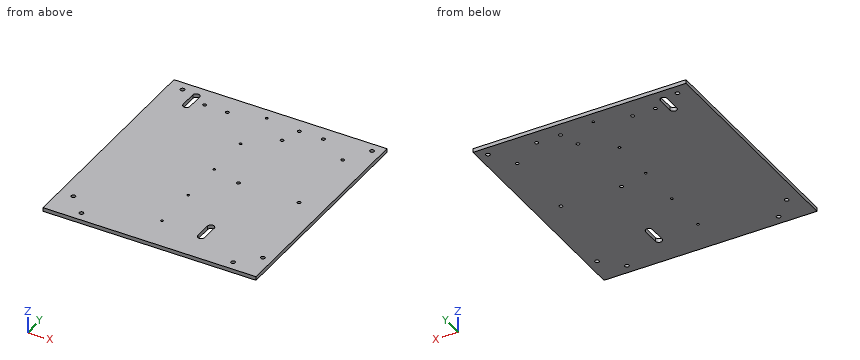
Autodesk Inventor part; units mm, degrees
ref_plane "YZ Plane" through (0, 0, 0) normal (1, 0, 0) x (0, 1, 0)
ref_plane "XZ Plane" through (0, 0, 0) normal (0, 1, 0) x (-1, 0, 0)
ref_plane "XY Plane" through (0, 0, 0) normal (0, 0, 1) x (1, 0, 0)
sketch "Sketch1" plane through (0, 0, 0) normal (0, 0, 1) x (1, 0, 0)
  line L0 (-140.5, -150) -> (140.5, -150)
  line L1 (140.5, -150) -> (140.5, 150)
  line L2 (140.5, 150) -> (-140.5, 150)
  line L3 (-140.5, 150) -> (-140.5, -150)
  line L4 (-140.5, -150) -> (140.5, 150) construction
  line L5 (140.5, -150) -> (-140.5, 150) construction
  point P0 (0, 0)
  dimension "d0" = 300
  dimension "d1" = 281
extrude "Extrusion1" add sketch "Sketch1" along normal blind 5
sketch "Sketch5" plane through (0, 0, 5) normal (0, 0, 1) x (1, 0, 0)
  line L0 (-140.5, -150) -> (140.5, -150)
  line L1 (140.5, -150) -> (140.5, 150)
  line L2 (140.5, 150) -> (-140.5, 150)
  line L3 (-140.5, 150) -> (-140.5, -150)
  line L4 (-122, -112.5) -> (128, -112.5) construction
  line L5 (128, -112.5) -> (128, 137.5) construction
  line L6 (128, 137.5) -> (-122, 137.5) construction
  line L7 (-122, 137.5) -> (-122, -112.5) construction
  line L8 (-122, -112.5) -> (128, 137.5) construction
  line L9 (128, -112.5) -> (-122, 137.5) construction
  circle A0 centre (-122, 137.5) radius 2.7
  circle A1 centre (128, 137.5) radius 2.7
  circle A2 centre (128, -112.5) radius 2.7
  circle A3 centre (-122, -112.5) radius 2.7
  circle A4 centre (-97, -137.5) radius 2.7
  circle A5 centre (103, -137.5) radius 2.7
  point P0 (0, 0)
  point P1 (3, 12.5)
  dimension "d34" = 18.5
  dimension "d35" = 37.5
  dimension "d36" = 12.5
  dimension "d37" = 5.4
  dimension "d38" = 12.5
  dimension "d39" = 37.5
  dimension "d40" = 43.5
  dimension "d83" = 12.5
extrude "Extrusion5" cut sketch "Sketch5" against normal through all contours A0 | A1 | A2 | A3 | A4 | A5
sketch "Sketch6" plane through (0, 0, 5) normal (0, 0, 1) x (1, 0, 0)
  line L0 (-140.5, -150) -> (140.5, -150)
  line L1 (140.5, -150) -> (140.5, 150)
  line L2 (-140.5, 150) -> (-140.5, -150)
  line L3 (-17, -110) -> (-2, -110) construction
  line L4 (-2, -110) -> (-2, 140) construction
  line L5 (-2, 140) -> (-17, 140) construction
  line L6 (-17, 140) -> (-17, -110) construction
  line L7 (-17, -110) -> (-2, 140) construction
  line L8 (-2, -110) -> (-17, 140) construction
  circle A0 centre (-9.5, 15) radius 1.6
  circle A1 centre (-9.5, 75) radius 1.6
  circle A2 centre (-9.5, 135) radius 1.6
  circle A3 centre (-9.5, -45) radius 1.6
  circle A4 centre (-9.5, -105) radius 1.6
  line L9 (-9.5, -105) -> (-9.5, -45) construction
  line L10 (-9.5, -45) -> (-9.5, 15) construction
  line L11 (-9.5, 15) -> (-9.5, 75) construction
  line L12 (-9.5, 75) -> (-9.5, 135) construction
  line L13 (115.5, -150) -> (-134.5, -150) construction
  line L14 (-134.5, -150) -> (-134.5, 62.3779) construction
  line L15 (-134.5, 62.3779) -> (115.5, 62.3779) construction
  line L16 (115.5, 62.3779) -> (115.5, -150) construction
  line L17 (-9.5, 62.3779) -> (-9.5, 15) construction
  point P0 (0, 0)
  dimension "d43" = 250
  dimension "d44" = 15
  dimension "d45" = 60
  dimension "d46" = 3.2
  dimension "d47" = 6
  dimension "d48" = 25
  dimension "d49" = 40
extrude "Extrusion6" cut sketch "Sketch6" against normal through all
sketch "Sketch7" plane through (0, 0, 0) normal (0, 0, -1) x (-1, 0, 0)
  circle A0 centre (9.5, 135) radius 1.6
  circle A1 centre (122, 137.5) radius 2.7
  circle A2 centre (-128, 137.5) radius 2.7
  line L0 (140.5, -150) -> (-140.5, -150)
  line L1 (140.5, 150) -> (140.5, -150)
  line L2 (-140.5, 150) -> (140.5, 150)
  line L3 (-140.5, -150) -> (-140.5, 150)
  line L4 (-53, -125) -> (-103, -125) construction
  line L5 (-103, -125) -> (-103, -74) construction
  line L6 (-103, -74) -> (-53, -74) construction
  line L7 (-53, -74) -> (-53, -125) construction
  line L8 (94.5, 150) -> (44.5, 150) construction
  line L9 (44.5, 150) -> (44.5, 96) construction
  line L10 (44.5, 96) -> (94.5, 96) construction
  line L11 (94.5, 96) -> (94.5, 150) construction
  circle A3 centre (54.5, 123) radius 2.2
  circle A4 centre (84.5, 123) radius 2.2
  line L12 (-45.5, -88.5) -> (-45.5, -110.5) construction
  line L13 (-50, -88.5) -> (-50, -110.5)
  line L14 (-41, -110.5) -> (-41, -88.5)
  arc A5 (-41, -88.5) -> (-50, -88.5) centre (-45.5, -88.5) ccw
  arc A6 (-50, -110.5) -> (-41, -110.5) centre (-45.5, -110.5) ccw
  line L15 (-45.5, -99.5) -> (-103, -99.5) construction
  line L16 (69.5, 96) -> (69.5, 144) construction
  line L17 (102, 134) -> (102, 112) construction
  line L18 (97.5, 134) -> (97.5, 112)
  line L19 (106.5, 112) -> (106.5, 134)
  arc A7 (106.5, 134) -> (97.5, 134) centre (102, 134) ccw
  arc A8 (97.5, 112) -> (106.5, 112) centre (102, 112) ccw
  line L20 (-73.3625, 150) -> (-30.5, 150) construction
  line L21 (-30.5, 150) -> (-30.5, 124.9969) construction
  line L22 (-30.5, 124.9969) -> (-73.3625, 124.9969) construction
  line L23 (-73.3625, 124.9969) -> (-73.3625, 150) construction
  circle A9 centre (-67.8063, 130.5531) radius 2.286
  circle A10 centre (-36.0563, 130.5531) radius 2.286
  line L24 (-108, 4.9969) -> (-28, 4.9969) construction
  line L25 (-28, 4.9969) -> (-28, 104.9969) construction
  line L26 (-28, 104.9969) -> (-108, 104.9969) construction
  line L27 (-108, 104.9969) -> (-108, 4.9969) construction
  line L28 (-108, 4.9969) -> (-28, 104.9969) construction
  line L29 (-28, 4.9969) -> (-108, 104.9969) construction
  circle A11 centre (-108, 104.9969) radius 2.2
  circle A12 centre (-28, 104.9969) radius 2.2
  circle A13 centre (-28, 4.9969) radius 2.2
  circle A14 centre (-108, 4.9969) radius 2.2
  point P0 (0, 0)
  point P1 (102, 123)
  point P2 (-68, 54.9969)
  dimension "d52" = 50
  dimension "d53" = 51
  dimension "d54" = 25
  dimension "d55" = 54
  dimension "d56" = 50
  dimension "d57" = 30
  dimension "d58" = 4.4
  dimension "d59" = 10
  dimension "d60" = 27
  dimension "d61" = 37.5
  dimension "d62" = 22
  dimension "d63" = 9
  dimension "d64" = 3
  dimension "d65" = 60
  dimension "d66" = 3
  dimension "d67" = 15.5
  dimension "d68" = 31.75
  dimension "d69" = 42.8625
  dimension "d70" = 5.5563
  dimension "d71" = 25.0031
  dimension "d72" = 5.5563
  dimension "d73" = 4.572
  dimension "d74" = 35
  dimension "d75" = 40
  dimension "d76" = 100
  dimension "d77" = 80
  dimension "d78" = 4.4
  dimension "d79" = 20
  dimension "d80" = 20
  dimension "d84" = 72.6937
  dimension "d85" = 19.4469
extrude "Extrusion7" cut sketch "Sketch7" against normal through all contours A3 | A4 | A5 L14 A6 L13 | A7 L19 A8 L18 | A9 | A10 | A11 | A12 | A13 | A14
equation "\"d59\" = -0.5 * d57 + 0.5 * d56"
equation "\"d60\" = 0.5 * d55"
equation "\"d72\" = -0.5 * d68 + 0.5 * d69"
properties part number "NewBackPlate"
The model under review builds one solid part; all positions refer to its coordinate system, in mm. Round coordinates to 2 decimals unless told otherwise and drop trailing zeros. Order: outer loops, then holes, each group sorted by start corner. A loop starts at its lowest first (then second) coordinate and runs counter-clockwise, first axis right, second up. Notation, with made-up numbers: (-26.75, 40) -> (-4.75, 40) arc R12 ccw to (-4.75, 47) -> close; hole circle Ø2 at (-34.5, -9.5). An arc over 180 degrees is marked (long way). Return JSON: item names as keys, results as strings.
1. Take a section at A-A (x = 45.5). Write out the cut boundary in (y, z).
Answer block:
{"outline": "(-150, 0) -> (-115, 0) -> (-115, 5) -> (-150, 5) -> close; (-84, 0) -> (150, 0) -> (150, 5) -> (-84, 5) -> close"}
2. For L1, parallel to Y at x = -97, z = 1.6; L2, parallel to X at y = 121, z = 2.8; L3, parallel to Y at x = 108, z = 4, list the stretches that pass through material, from the lowest coordinate up. Write a range as [from, to].
Answer block:
{"L1": "y = [-150, -140.2], [-134.8, 150]", "L2": "x = [-140.5, -106.5], [-97.5, -85.42], [-83.58, -55.42], [-53.58, 140.5]", "L3": "y = [-150, 2.8], [7.2, 102.8], [107.2, 150]"}
3. Insertion check: P1, Ø6, axis at x = 36.06, y = 130.55, coming from the +Z side; P2, Ø1.9, axis at x = -9.5, y = 75, coming from the +Z side. Each pin has a flat end and moves straight along its axis. Give the tip position at first contact, or say it passes through.
Answer block:
{"P1": "stops at z = 5", "P2": "passes through"}
